Autodesk Inventor part; units mm, degrees
ref_plane "YZ Plane" through (0, 0, 0) normal (1, 0, 0) x (0, 1, 0)
ref_plane "XZ Plane" through (0, 0, 0) normal (0, 1, 0) x (-1, 0, 0)
ref_plane "XY Plane" through (0, 0, 0) normal (0, 0, 1) x (1, 0, 0)
sketch "Sketch1" plane through (0, 0, 0) normal (0, 0, 1) x (1, 0, 0)
  circle A0 centre (0, 0) radius 2.3813
  dimension "d0" = 4.7625
extrude "Extrusion1" add sketch "Sketch1" along normal blind 38.1
sketch "Sketch2" plane through (0, 0, 38.1) normal (0, 0, 1) x (1, 0, 0)
  circle A0 centre (0, 0) radius 2.3813
  arc A1 (-3.81, 0) -> (3.81, 0) centre (0, 0) ccw
  line L0 (-3.81, 0) -> (3.81, 0)
  arc A2 (3.81, 0) -> (-3.81, 0) centre (0, 0) ccw
  dimension "d3" = 7.62
revolve "Revolution1" add sketch "Sketch2" angle 180 about axis through (-3.81, 0, 38.1) along (1, 0, 0) picked at (0.5941, 0.5264) contours L0 A0 | A0 L0 A2
thread "Thread1"
chamfer "Chamfer1" distance 0.381 angle 45 1 edges at (-2.3813, 0, 0)
properties part number "screw"
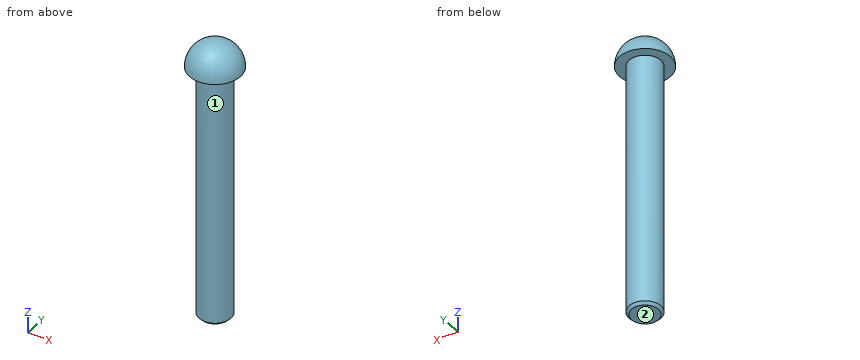
Verification items for the finished model (mm, model axes). Face numbers are marked on the shaded views. A direction names the side the tool comes from. Round coordinates to 2 decimals unless told otherwise and drop trailing zeros. Order: outer loops, then holes, each group sorted by start corner. A loop starts at its lowest first (then second) coordinate and runs counter-clockwise, first axis right, second up. Notation, with made-up numbers: (45.25, 44.25) -> (61.25, 44.25) arc R34 ccw to (61.25, 78.25) -> close; hole circle Ø7 at (-34.75, 75.25). An arc over 180 degrees is marked (long way). Put each result on its own line as item: value.
1) Section check C-C (z = 9). Record the cut outline in (x, y).
Final values:
outline: circle Ø4.76 at (0, 0)
2) Depth check by flat-ended pin: pin 1 (4 mm diameter, centred on y = 0.5, z = 12.5, fed in from +X); pin 2 (1 mm diameter, centred on y = 2.5, z = 33, fed in from +X); pin 3 (1.5 mm diameter, centred on x = 0.5, z = 29.5, fed in from -Y). Enter the tip coordinate at first touch or a pass-through.
Final values:
pin 1: stops at x = 2.38
pin 2: stops at x = 1.29
pin 3: stops at y = -2.38
3) Section check A-A (x = 0). Record the cut outline in (y, z), then the cut area to 3 significant figures.
Final values:
outline: (-3.81, 38.1) -> (-2.38, 38.1) -> (-2.38, 0.38) -> (-2, 0) -> (2, 0) -> (2.38, 0.38) -> (2.38, 38.1) -> (3.81, 38.1) arc R3.81 ccw to start
area: 204 mm^2
4) Section check D-D (x = -3). Record the cut outline in (y, z).
Final values:
outline: (-2.35, 38.1) -> (2.35, 38.1) arc R2.35 ccw to start
5) Material ranges on line 1 (Y direction, x = -1, z = 3); line 2 (Y direction, x = 0, z = 34.5); line 3 (X direction, y = -2, z = 20), recorded low to high.
Final values:
line 1: y = -2.16 to 2.16
line 2: y = -2.38 to 2.38
line 3: x = -1.29 to 1.29
6) Set-up check for the marked faces 1 and 2: record each of +Z, -Z, +X, -X, +Y, -Y from which the full face is reachable in a straight line by a thin tool's end or side.
Final values:
face 1: -Z
face 2: -Z, +X, -X, +Y, -Y
